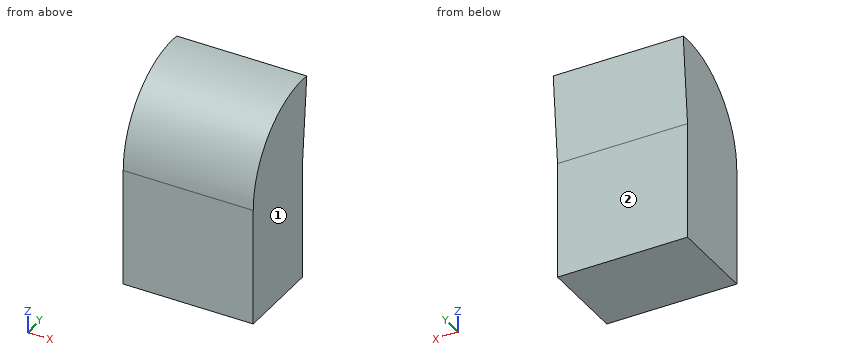
from build123d import *

# Parameters (mm, degrees)
F2_W     = 914.4
F2_H     = 609.6
F3_DEPTH = 825.5
F4_W     = 914.4
F4_H     = 609.6
F5_ANGLE = 95


# Not quite as in the source:
# - a variable given as a bare number and used for a length is read in inches; the dataset says mm whatever the document's units were


with BuildPart() as f3:
    # F2 (on Top) → F3 (new body)
    with BuildSketch(Plane.XY):
        Rectangle(F2_W, F2_H)
    extrude(amount=F3_DEPTH)

    # F4 (on face) → F5 (revolve)
    with BuildSketch(Plane.XY.offset(825.5)):
        Rectangle(F4_W, F4_H)
    revolve(axis=Axis((0, 304.8, 825.5), (-1, 0, 0)), revolution_arc=F5_ANGLE)


solid = f3.part
Design review of the part built by this model. Coordinates are the model's own, in mm. Face numbers are marked on the shaded views. A direction names the side the tool comes from. Round coordinates to 2 decimals unless told otherwise and drop trailing zeros. Write each loop counter-clockwise with the first axis right and the second up, starting at its lowest first coordinate (ties: lowest second). Pieces come first, ordered by that corner, then holes.
Item 1: Consider section B-B on z = 440.5. Give the boundary of the cut face in (x, y), and give its area (3 significant figures).
Item 2: Consider section C-C on y = 22. Give the boundary of the cut face in (x, z), and give its area (3 significant figures).
Item 3: Consider section A-A on x = -67. Give the boundary of the cut face in (y, z).
Item 4: For pin 1 Ø6 at (x, z) = (-28.5, 243.5) entering from +Y, flat-tipped, find the tip position at first contact; note if it passes through.
Item 5: Wall thickness on L1, parallel to Y at x = 370.5, z = 393.5; L2, parallel to Z at x = 301.5, y = 222; L3, parallel to Z at x = -284.5, y = 126: over which ranges is each line inside the solid? List them lowest first.
Item 6: For the marked faces 1 and 2, list the 3-axis set-ups (+Z, -Z, +X, -X, +Y, -Y) from which the entire face can be reached by the end or side of a thin tool; tool diameter is ignored.
Check values:
1. outline: (-457.2, -304.8) - (457.2, -304.8) - (457.2, 304.8) - (-457.2, 304.8) - close
1. area: 557,000 mm2
2. outline: (-457.2, 0) - (457.2, 0) - (457.2, 1365.53) - (-457.2, 1365.53) - close
2. area: 1,250,000 mm2
3. outline: (-304.8, 0) - (304.8, 0) - (304.8, 825.5) - (357.93, 1432.78) arc R609.6 ccw to (-304.8, 825.5) - close
4. pin 1: stops at y = 304.8
5. L1: y = -304.8 to 304.8
5. L2: z = 0 to 1429.45
5. L3: z = 0 to 1408.29
6. face 1: +Z, -Z, +X, +Y, -Y
6. face 2: -Z, +X, -X, +Y
